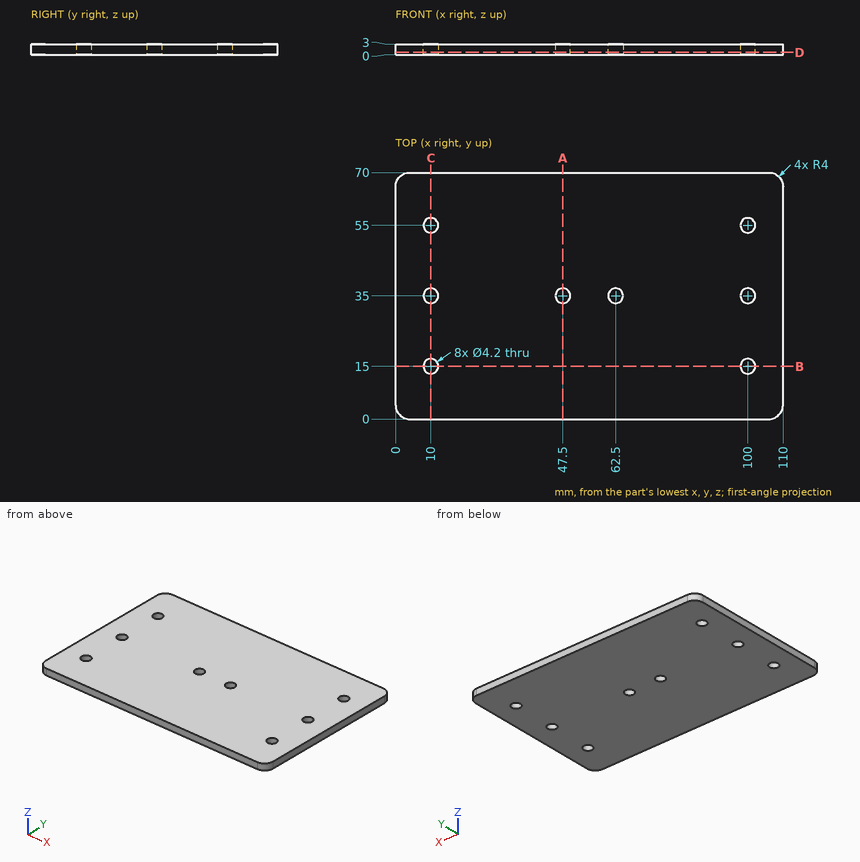
Part print with two shaded views. Sizes in mm from the minimum x, y, z corner. Round coordinates to 2 decimals unless told otherwise and drop trailing zeros. Loops run counter-clockwise (first coordinate to the right, second up) from the corner with the lowest first, then second, coordinate; pieces in that order, holes last. Notation, with made-up numbers: (85, 34.5) - (89, 34.5) arc R9 ccw to (89, 49.5) - close; hole circle Ø8 at (-18.75, -12.5). An arc over 180 degrees is marked (long way). Put each result on its own line as item: value.
1. Pin check, flat tip, straight feed: P1, Ø5.5, axis at x = 100, y = 15, coming from the +Z side. Stop position of the tip, or through.
Geometry check:
P1: z = 3
2. Wall check: line 1 (Y direction, x = 10, z = 1.45); line 2 (X direction, y = 3.5, z = 0.7). Give the ranges that are in metal, low to high.
Geometry check:
line 1: 0 to 12.9, 17.1 to 32.9, 37.1 to 52.9, 57.1 to 70
line 2: 0.03 to 109.97
3. Slice it at B-B on y = 15. List the corners of the cut face in (x, z).
Geometry check:
outline: (0, 0) - (7.9, 0) - (7.9, 3) - (0, 3) - close; (12.1, 0) - (97.9, 0) - (97.9, 3) - (12.1, 3) - close; (102.1, 0) - (110, 0) - (110, 3) - (102.1, 3) - close
4. Slice it at D-D on z = 0.6. Give the number of separate pieces and of enclosed holes in the cut face, and give its area (3 significant figures).
Geometry check:
separate pieces: 1
enclosed holes: 8
area: 7,580 mm²
5. Slice it at C-C on x = 10. List the corners of the cut face in (y, z).
Geometry check:
outline: (0, 0) - (12.9, 0) - (12.9, 3) - (0, 3) - close; (17.1, 0) - (32.9, 0) - (32.9, 3) - (17.1, 3) - close; (37.1, 0) - (52.9, 0) - (52.9, 3) - (37.1, 3) - close; (57.1, 0) - (70, 0) - (70, 3) - (57.1, 3) - close
6. Slice it at A-A on x = 47.5. List the corners of the cut face in (y, z).
Geometry check:
outline: (0, 0) - (32.9, 0) - (32.9, 3) - (0, 3) - close; (37.1, 0) - (70, 0) - (70, 3) - (37.1, 3) - close
